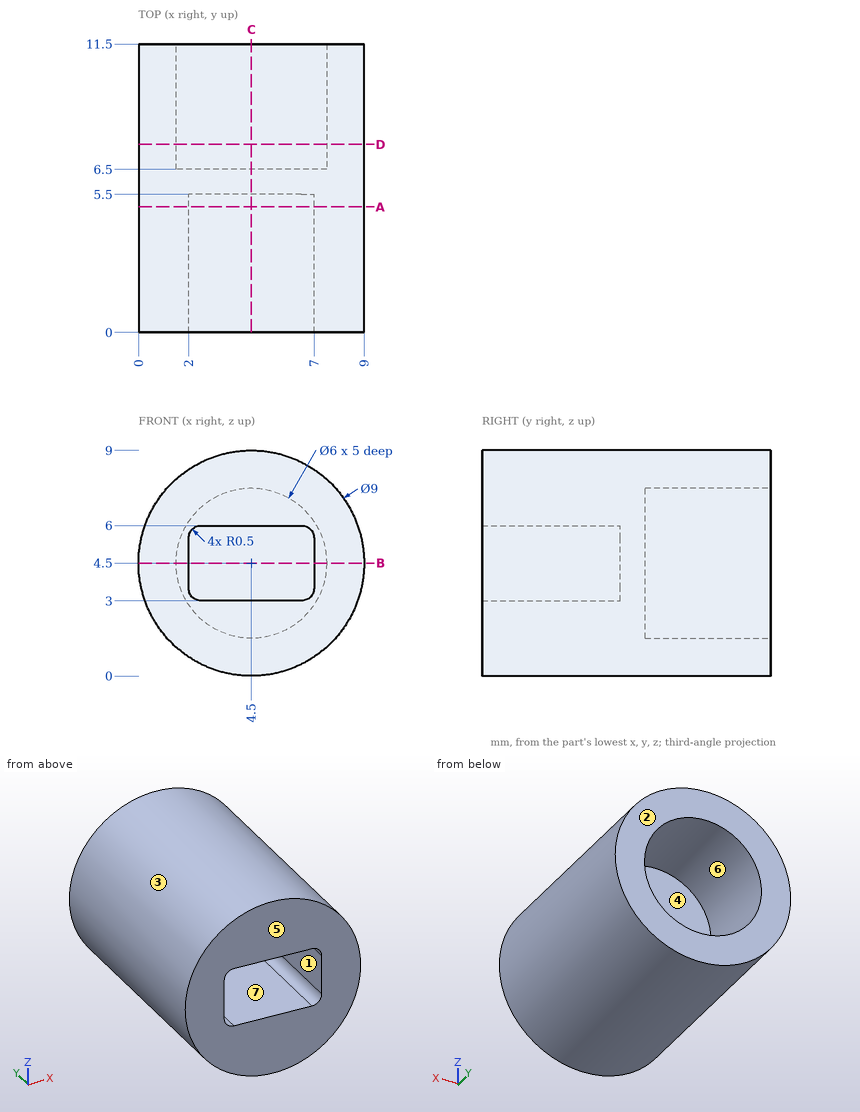
Verification items for this drawing (mm, ordinates from the low corner). A direction names the side the tool comes from. Coordinates: 2 decimals unless noted, no trailing zeros. Loops run counter-clockwise (first coordinate to the right, second up) from the corner with the lowest first, then second, coordinate; pieces in that order, holes last. Notation, with made-up numbers: (72.5, 24.5) - (104.5, 24.5) arc R31 ccw to (104.5, 62.5) - close; hole circle Ø8 at (35, -34.75). An arc over 180 degrees is marked (long way). Use one line per item in the form item = value. Start each with the question number.
Item 1: Section check C-C, the plane x = 4.5. Enter the section's corners in (y, z), and give its area (3 significant figures).
Item 2: Thickness scan on probe 1 along Z at (x, y) = (4.5, 9); probe 2 along X at (y, z) = (8.25, 7.25). Record the ranges inside material, lowest first.
Item 3: Section check A-A, the plane y = 5. Enter the section's corners in (x, z), and give its area (3 significant figures).
Item 4: Mould release check, pull along Z, two halves, no side actions. Record for the marked faces 1, 2, 3 and 4: +Z half, -Z half, draft (parallel to the pull), parting line (faces both ways), or undercut.
Item 5: Section check D-D, the plane y = 7.5. Enter the section's corners in (x, z), and give its area (3 significant figures).
Item 6: Section check B-B, the plane z = 4.5. Enter the section's corners in (x, y), and give its area (3 significant figures).
Item 7: Gauge pin test, flat ends, axial feed: pin 1 (3 mm diameter, centred on x = 3.5, z = 5.5, fed in from -Y); pin 2 (2 mm diameter, centred on y = 4, z = 8, fed in from -X); pin 3 (1.5 mm diameter, centred on y = 2, z = 5.5, fed in from +X). Record the tip position at first contact, or that the pin passes through.
Item 8: Tool access check on the marked faces 5, 6 and 7. Record the directions out of +Z, -Z, +X, -X, +Y, -Y that give a thin tool (end or side, any length) a straight path to the whole face; none if there is none.
Computed:
q1.outline = (0, 0) - (11.5, 0) - (11.5, 1.5) - (6.5, 1.5) - (6.5, 7.5) - (11.5, 7.5) - (11.5, 9) - (0, 9) - (0, 6) - (5.5, 6) - (5.5, 3) - (0, 3) - close
q1.area = 57.0 mm2
q2.probe_1 = 0 to 1.5, 7.5 to 9
q2.probe_2 = 0.94 to 3.3, 5.7 to 8.06
q3.outline = circle Ø9 at (4.5, 4.5); hole (2, 3.5) arc R0.5 ccw to (2.5, 3) - (6.5, 3) arc R0.5 ccw to (7, 3.5) - (7, 5.5) arc R0.5 ccw to (6.5, 6) - (2.5, 6) arc R0.5 ccw to (2, 5.5) - close
q3.area = 48.8 mm2
q4.face_1 = undercut
q4.face_2 = draft
q4.face_3 = parting line
q4.face_4 = undercut
q5.outline = circle Ø9 at (4.5, 4.5); hole circle Ø6 at (4.5, 4.5)
q5.area = 35.3 mm2
q6.outline = (0, 0) - (2, 0) - (2, 5.5) - (7, 5.5) - (7, 0) - (9, 0) - (9, 11.5) - (7.5, 11.5) - (7.5, 6.5) - (1.5, 6.5) - (1.5, 11.5) - (0, 11.5) - close
q6.area = 46.0 mm2
q7.pin_1 = 0
q7.pin_2 = 0.76
q7.pin_3 = 8.99
q8.face_5 = +Z, -Z, +X, -X, -Y
q8.face_6 = +Y
q8.face_7 = -Y
